from build123d import *

# Parameters (mm, degrees)
SKETCH4_R             = 4.5339
SKETCH4_R_2           = 4.37515
CUT_EXTRUDE2_DEPTH    = 4.064
CUT_EXTRUDE1_DEPTH    = 4.064
CIRPATTERN1_COUNT     = 14
SKETCH6_R             = 1.5875
CUT_EXTRUDE3_DEPTH    = 12.02520933
CUT_EXTRUDE4_DEPTH    = 1.016
SKETCH11_R            = 6.731
CUT_EXTRUDE6_DEPTH    = 2.54
SKETCH13_R            = 9.525
CUT_EXTRUDE7_DEPTH    = 12.262802402
BOSS_EXTRUDE2_START   = -4.064
SKETCH17_R            = 1.5875
SKETCH17_R_2          = 1.4732
BOSS_EXTRUDE2_DEPTH   = 4.064
BOSS_EXTRUDE1_START   = 2.54
SKETCH12_R            = 1.4732
BOSS_EXTRUDE1_DEPTH   = 2.54
F_4_CLEARANCE_HOLE1_D = 2.9464


with BuildPart() as part:
    # Sketch1 → Revolve1 (revolve)
    with BuildSketch(Plane.XY, mode=Mode.PRIVATE) as revolve1_sk:
        with BuildLine():
            Line((-5.5626, 1.5875), (5.5626, 1.5875))
            Line((5.5626, 1.5875), (5.5626, 6.731))
            Line((5.5626, 6.731), (5.0419, 6.731))
            ThreePointArc((5.0419, 6.731), (4.654552953, 5.958878742), (4.5212, 5.1054))
            Line((4.5212, 5.1054), (4.5212, 4.5339))
            Line((4.5212, 4.5339), (0.4572, 4.5339))
            Line((0.4572, 4.5339), (0.4572, 5.6769))
            Line((0.4572, 5.6769), (-0.5969, 6.731))
            Line((-0.5969, 6.731), (-5.5626, 6.731))
            Line((-5.5626, 6.731), (-5.5626, 1.5875))
        make_face()
    revolve(revolve1_sk.sketch.rotate(Axis((-5.5626, 0, 0), (1, 0, 0)), 90), axis=Axis((-5.5626, 0, 0), (1, 0, 0)))

    # Sketch4 → Cut-Extrude2 (cut)
    with BuildSketch(Plane(origin=(0.4572, 0, 0), x_dir=(0, 0, -1), z_dir=(1, 0, 0))):
        Circle(SKETCH4_R)
        Circle(SKETCH4_R_2, mode=Mode.SUBTRACT)
    extrude(amount=CUT_EXTRUDE2_DEPTH, mode=Mode.SUBTRACT)

    # Sketch3 → Cut-Extrude1 (cut)
    with BuildSketch(Plane(origin=(0.4572, 0, 0), x_dir=(0, 0, -1), z_dir=(1, 0, 0))):
        with BuildLine():
            Line((-0.641613493, 4.327848154), (-0.345249615, 3.692293767))
            Line((-0.345249615, 3.692293767), (0.345249615, 3.692293767))
            Line((0.345249615, 3.692293767), (0.641613493, 4.327848154))
            ThreePointArc((0.641613493, 4.327848154), (0, 4.37515), (-0.641613493, 4.327848154))
        make_face()
    cut_extrude1 = extrude(amount=CUT_EXTRUDE1_DEPTH, mode=Mode.SUBTRACT)

    # CirPattern1: Cut-Extrude1 ×14 about axis
    cirpattern1_axis = Axis((0, 0, 0), (1, 0, 0))
    for i in range(1, CIRPATTERN1_COUNT):
        add(cut_extrude1.rotate(cirpattern1_axis, i * 360 / CIRPATTERN1_COUNT), mode=Mode.SUBTRACT)

    # Sketch6 → Cut-Extrude3 (cut, through all)
    with BuildSketch(Plane(origin=(0, 0, 0), x_dir=(1, 0, 0), z_dir=(0, 1, 0))):
        with Locations(Location((-2.5527, 0, 0), (0, 0, 90))):
            Circle(SKETCH6_R)
    extrude(amount=CUT_EXTRUDE3_DEPTH, mode=Mode.SUBTRACT)

    # Sketch11 → Cut-Extrude6 (cut)
    with BuildSketch(Plane.ZY.offset(-4.5212)):
        Circle(SKETCH11_R)
    extrude(amount=-CUT_EXTRUDE6_DEPTH, mode=Mode.SUBTRACT)


with BuildPart() as body_2:
    # Sketch7 → Revolve2 (revolve)
    with BuildSketch(Plane.XY, mode=Mode.PRIVATE) as revolve2_sk:
        Polygon((-3.7211, 6.731), (-2.5527, 6.731), (-2.5527, 1.9685), (-3.7211, 1.9685), (-3.9751, 2.2225), (-3.9751, 6.477), align=None)
    revolve(revolve2_sk.sketch.rotate(Axis((-2.5527, 1.9685, 0), (0, 1, 0)), 270), axis=Axis((-2.5527, 1.9685, 0), (0, 1, 0)))

    # Sketch8 → Cut-Extrude4 (cut)
    with BuildSketch(Plane(origin=(0, 6.731, 0), x_dir=(1, 0, 0), z_dir=(0, 1, 0))):
        Polygon((-2.5527, 0.821223023), (-3.2639, 0.410611511), (-3.2639, -0.410611511), (-2.5527, -0.821223023), (-1.8415, -0.410611511), (-1.8415, 0.410611511), align=None)
    extrude(amount=-CUT_EXTRUDE4_DEPTH, mode=Mode.SUBTRACT)


with BuildPart() as cut_extrude7_tool:
    # Sketch13 → Cut-Extrude7 (new, through all)
    with BuildSketch(Plane(origin=(0.4572, 0, 0), x_dir=(0, 0, -1), z_dir=(1, 0, 0))):
        Circle(SKETCH13_R)
    extrude(amount=-CUT_EXTRUDE7_DEPTH)


with BuildPart() as part_1:
    add(part.part)

    # Cut-Extrude7: cut by cut_extrude7_tool
    add(cut_extrude7_tool.part, mode=Mode.SUBTRACT)

    # Sketch17 → Boss-Extrude2 (add)
    with BuildSketch(Plane.ZY.offset(-0.4572).offset(BOSS_EXTRUDE2_START)):
        Circle(SKETCH17_R)
        Circle(SKETCH17_R_2, mode=Mode.SUBTRACT)
    extrude(amount=BOSS_EXTRUDE2_DEPTH)

    # Sketch12 → Boss-Extrude1 (add)
    with BuildSketch(Plane(origin=(4.5212, 0, 0), x_dir=(0, 0, -1), z_dir=(1, 0, 0)).offset(BOSS_EXTRUDE1_START)):
        with BuildLine():
            Line((6.35, 0), (6.35, -44.45))
            Line((6.35, -44.45), (-6.35, -44.45))
            Line((-6.35, -44.45), (-6.35, 0))
            ThreePointArc((-6.35, 0), (0, 6.35), (6.35, 0))
        make_face()
        with Locations(Location((0, 0, 0), (0, 0, 180))):
            Circle(SKETCH12_R, mode=Mode.SUBTRACT)
    extrude(amount=-BOSS_EXTRUDE1_DEPTH)

    # #4 Clearance Hole1 (through all)
    with Locations(Plane(origin=(7.0612, 0, 0), x_dir=(0, 0, -1), z_dir=(1, 0, 0))):
        with Locations((0, -31.75), (0, -38.1)):
            Hole(F_4_CLEARANCE_HOLE1_D / 2)


with BuildPart() as body_2_1:
    add(body_2.part)

    # Cut-Extrude7: cut by cut_extrude7_tool
    add(cut_extrude7_tool.part, mode=Mode.SUBTRACT)


solid = part_1.part
The listing builds one solid part. Answer for the finished solid, in the listing's coordinates (mm). Round coordinates to 2 decimals unless told otherwise and drop trailing zeros. Order: outer loops, then holes, each group sorted by start corner. A loop starts at its lowest first (then second) coordinate and runs counter-clockwise, first axis right, second up. Notation, with made-up numbers: M 65.5,-35.75 L 124.5,-35.75 A33 ccw 124.5,-4.75 Z; hole C -7,86.5 d2. An arc over 180 degrees is marked long. Answer in a Markdown table with one row per item. Add a question column.
1) Consider line 1 along Y through (x, z) = (5.45, 0); line 2 along Y through (x, z) = (3.25, 4); line 3 along Y through (x, z) = (3.5, 0). Determine where each line is inside the solid, lowest interval first. Write a range as from..to.
2) The part is cut by section A-A on y = -31.75. Determine the outline of the cut face in (x, z).
3) The part is cut by section D-D on z = 5.25. Determine the outline of the cut face in (x, y), plus the area to 3 significant figures.
4) The part is cut by section C-C on y = -11. Determine the outline of the cut face in (x, z).
5) Determine the mould class of faces 1 (the face through (6, -23, 6.35)), 2 (the face through (5.77, -36.64, -0.19)), 3 (the face through (6, -22, -6.35)), 4 (the face through (5.77, -33.19, -0.32)) for opening direction Z: pulls with the +Z half, pulls with the -Z half, needs draft (parallel to the pull), parting line crosses it, or undercut.
6) The part is cut by section B-B on x = 6. Determine the outline of the cut face in (y, z).
7) Flat-ended cylindrical pins translate along their axes: pin 1 Ø1 at (x, z) = (5, -1) entering from +Y; pin 2 Ø1 at (x, z) = (3.5, 4.5) entering from +Y; pin 3 Ø0.6 at (x, z) = (2.5, 0) entering from +Y. Find the tip coordinate at first contact, or state that the pin passes through.
Findings below:
| question | item | result |
|---|---|---|
| 1 | line 1 | y = -44.45..-39.57, -36.63..-33.22, -30.28..-1.47, 1.47..6.35 |
| 1 | line 2 | y = -1.77..-1.53, -0.42..0.42, 1.53..1.77 |
| 1 | line 3 | y = -3.69..-1.47, 1.47..3.69 |
| 2 | outline | M 4.52,-6.35 L 7.06,-6.35 L 7.06,-1.47 L 4.52,-1.47 Z; M 4.52,1.47 L 7.06,1.47 L 7.06,6.35 L 4.52,6.35 Z |
| 3 | outline | M 4.52,-44.45 L 7.06,-44.45 L 7.06,3.57 L 4.52,3.57 Z |
| 3 | area | 122 mm² |
| 4 | outline | M 4.52,-6.35 L 7.06,-6.35 L 7.06,6.35 L 4.52,6.35 Z |
| 5 | face 1 | pulls with the +Z half |
| 5 | face 2 | undercut |
| 5 | face 3 | pulls with the -Z half |
| 5 | face 4 | undercut |
| 6 | outline | M -44.45,-6.35 L 0,-6.35 A6.35 ccw 0,6.35 L -44.45,6.35 Z; hole C -38.1,0 d2.95; hole C -31.75,0 d2.95; hole C 0,0 d2.95 |
| 7 | pin 1 | stops at y = 6.33 |
| 7 | pin 2 | stops at y = 1.77 |
| 7 | pin 3 | stops at y = 3.69 |
